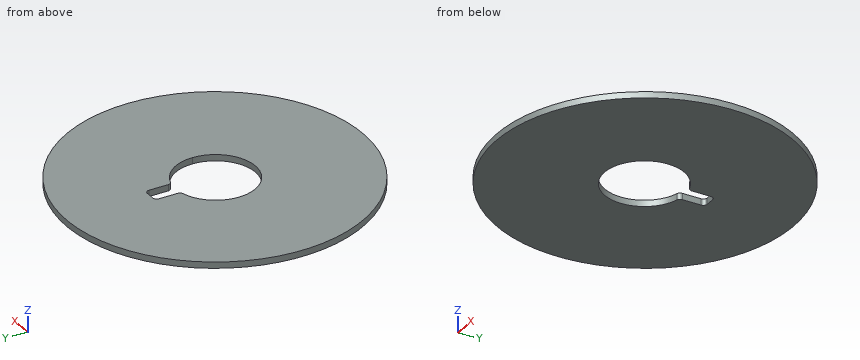
```python
from build123d import *

# Parameters (mm, degrees)
F0_R     = 19
F1_DEPTH = 0.8
F2_R     = 0.5


with BuildPart() as f1:
    # F0 (on Top) → F1 (new body)
    with BuildSketch(Plane.XY):
        Circle(F0_R)
        with BuildLine():
            ThreePointArc((1.1, 4.946329), (3.879108, 3.136336), (4.957492, 0))
            ThreePointArc((4.957492, 0), (-3.392645, -3.930217), (-1.1, 5.009312))
            Line((-1.1, 5.009312), (-1.1, 8.298009))
            Line((-1.1, 8.298009), (1.1, 8.298009))
            Line((1.1, 8.298009), (1.1, 4.946329))
        make_face(mode=Mode.SUBTRACT)
    extrude(amount=F1_DEPTH)

    # F2
    f2_edges = [f1.edges().sort_by_distance(p)[0] for p in [
        (1.1, 4.946329, 0.4),
        (1.1, 8.298009, 0.4),
        (-1.1, 8.298009, 0.4),
        (-1.1, 5.009312, 0.4),
    ]]
    fillet(f2_edges, radius=F2_R)


solid = f1.part
```
Input: part model. Units: mm. Frame: model coordinates. Coordinates: 2 decimals unless noted, no trailing zeros. Loops run counter-clockwise (first coordinate to the right, second up) from the corner with the lowest first, then second, coordinate; pieces in that order, holes last. Notation, with made-up numbers: (24.5, 31.5) -> (75.5, 31.5) arc R18 cw to (75.5, 55.5) -> close; hole circle Ø3 at (10.5, 14). An arc over 180 degrees is marked (long way). Use a Markdown table: item, result.
1) Cut plane A-A (z = 0.55). Return the cut outline in (x, y), then the cut area to 3 significant figures.
Results found:
| item | result |
|---|---|
| outline | circle Ø38 at (0, 0); hole (-1.47, 4.92) arc R5.1 ccw (long way) to (1.44, 4.85) arc R0.5 cw to (1.1, 5.32) -> (1.1, 7.8) arc R0.5 ccw to (0.6, 8.3) -> (-0.6, 8.3) arc R0.5 ccw to (-1.1, 7.8) -> (-1.1, 5.41) arc R0.5 cw to start |
| area | 1,050 mm2 |
2) Cut plane D-D (x = -11). Return the cut outline in (y, z).
Results found:
| item | result |
|---|---|
| outline | (-15.49, 0) -> (15.49, 0) -> (15.49, 0.8) -> (-15.49, 0.8) -> close |
3) Cut plane C-C (y = -7.5). Return the cut outline in (x, z), then the cut area to 3 significant figures.
Results found:
| item | result |
|---|---|
| outline | (-17.46, 0) -> (17.46, 0) -> (17.46, 0.8) -> (-17.46, 0.8) -> close |
| area | 27.9 mm2 |
4) Contact query for a flat-ended pin moving along its axis: pin 1 (6 mm diameter, centred on x = -0.14, y = 0, fed in from +Z). Output: stop coordinate, or through.
Results found:
| item | result |
|---|---|
| pin 1 | passes through |
5) Material intervals for line 1 along Y through (x, z) = (-3, 0.35); line 2 along Y through (x, z) = (4, 0.2); line 3 along X through (y, z) = (6.5, 0.3), sorted ascending. Write a range as from..to.
Results found:
| item | result |
|---|---|
| line 1 | y = -18.76..-4.22, 4.22..18.76 |
| line 2 | y = -18.57..-2.97, 2.97..18.57 |
| line 3 | x = -17.85..-1.1, 1.1..17.85 |
6) Cut plane B-B (x = 0). Return the cut outline in (y, z).
Results found:
| item | result |
|---|---|
| outline | (-19, 0) -> (-5.1, 0) -> (-5.1, 0.8) -> (-19, 0.8) -> close; (8.3, 0) -> (19, 0) -> (19, 0.8) -> (8.3, 0.8) -> close |
